Check sheet for the modelled part. Datum: model origin and axes. Units: mm. Face numbers are marked on the shaded views. Round coordinates to 2 decimals unless told otherwise and drop trailing zeros. Order: outer loops, then holes, each group sorted by start corner. A loop starts at its lowest first (then second) coordinate and runs counter-clockwise, first axis right, second up.
Q1. Cross-section at B-B on y = 10.5. Record the cut outline in (x, z), then the cut area to 3 significant figures.
Q2. Scan lines: probe 1 along X at (y, z) = (-25.5, -4.25); probe 2 along Z at (x, y) = (26, 0); probe 3 along X at (y, z) = (36.5, -10.5). Record each from-to range of solid material in increasing order.
Q3. Depth check by flat-ended pin: P1, Ø1, axis at x = -37.5, y = 12.5, coming from the +Z side. Enter the tip coordinate at first touch or a pass-through.
Q4. Cross-section at C-C on x = 68. Record the cut outline in (y, z), then the cut area to 3 significant figures.
Q5. Mould release check, pull along X, two halves, no side actions. Record for the marked faces 1 and 2: +X half, -X half, draft (parallel to the pull), parting line (faces both ways), or undercut.
Q6. Cross-section at A-A on z = -7.25. Record the cut outline in (x, y).
from build123d import *

# Parameters (mm, degrees)
F1_DEPTH = 40
F2_R     = 1
F3_R     = 4


with BuildPart() as f1:
    # F0 (on Front) → F1 (new body, symmetric)
    with BuildSketch(Plane.XZ):
        Polygon((-99.5, 0), (-99.5, -13), (99.5, -13), (99.5, 0), (96.5, 0), (96.5, -10), (-96.5, -10), (-96.5, 0), align=None)
    extrude(amount=F1_DEPTH, both=True)

    # F2
    f2_edges = [f1.edges().sort_by_distance(p)[0] for p in [
        (-96.5, 0, -10),
        (96.5, 0, -10),
    ]]
    fillet(f2_edges, radius=F2_R)

    # F3
    f3_edges = [f1.edges().sort_by_distance(p)[0] for p in [
        (-99.5, 0, -13),
        (99.5, 0, -13),
    ]]
    fillet(f3_edges, radius=F3_R)


solid = f1.part
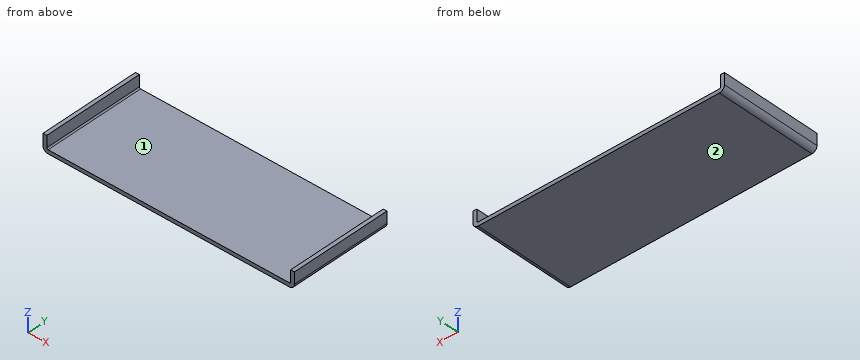
Results found:
1. outline: (-99.5, -9) arc R4 ccw to (-95.5, -13) - (95.5, -13) arc R4 ccw to (99.5, -9) - (99.5, 0) - (96.5, 0) - (96.5, -9) arc R1 cw to (95.5, -10) - (-95.5, -10) arc R1 cw to (-96.5, -9) - (-96.5, 0) - (-99.5, 0) - close
1. area: 651 mm2
2. probe 1: x = -99.5 to -96.5, 96.5 to 99.5
2. probe 2: z = -13 to -10
2. probe 3: x = -99.21 to 99.21
3. P1: stops at z = -10
4. outline: (-40, -13) - (40, -13) - (40, -10) - (-40, -10) - close
4. area: 240 mm2
5. face 1: undercut
5. face 2: draft
6. outline: (-99.5, -40) - (-96.5, -40) - (-96.5, 40) - (-99.5, 40) - close; (96.5, -40) - (99.5, -40) - (99.5, 40) - (96.5, 40) - close
